Can you work these out from the model? Positions are in its coordinate system, mm. Face numbers are marked on the shaded views. A direction names the side the tool comes from. Coordinates: 2 decimals unless noted, no trailing zeros. Order: outer loops, then holes, each group sorted by start corner. A loop starts at its lowest first (then second) coordinate and runs counter-clockwise, first axis right, second up. Notation, with made-up numbers: (77, 11.5) -> (107, 11.5) arc R22 cw to (107, 36.5) -> close; hole circle Ø8 at (41.25, 20). An arc over 180 degrees is marked (long way). Write item = value, one per line.
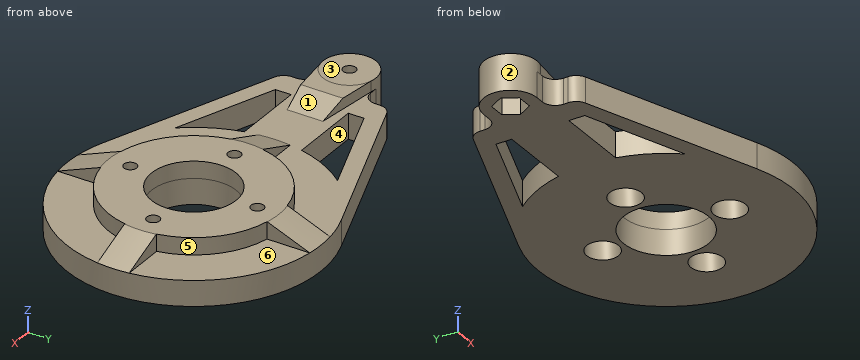
```python
from build123d import *
from OCP.BRepFilletAPI import BRepFilletAPI_MakeChamfer
from build123d.topology import SkipClean

# Parameters (mm, degrees)
SKETCH2_R           = 40
SKETCH2_R_2         = 20
BOSS_EXTRUDE1_DEPTH = 8
BOSS_EXTRUDE2_START = 12
SKETCH3_R           = 20
BOSS_EXTRUDE2_DEPTH = 12
SKETCH4_R           = 7.5
CUT_EXTRUDE1_DEPTH  = 10
SKETCH5_R           = 3
CUT_EXTRUDE2_DEPTH  = 29
BOSS_EXTRUDE3_DEPTH = 8
CHAMFER3_SIZE       = 8
CHAMFER3_SIZE_2     = 19.800694827
BOSS_EXTRUDE4_DEPTH = 12
FILLET1_R           = 6
CUT_EXTRUDE3_DEPTH  = 10
SKETCH9_R           = 3
CUT_EXTRUDE4_DEPTH  = 6
CUT_EXTRUDE5_START  = -22
CUT_EXTRUDE5_DEPTH  = 22
SKETCH12_R          = 12.5
SKETCH12_R_2        = 3
BOSS_EXTRUDE5_DEPTH = 5
BOSS_EXTRUDE6_DEPTH = 5
CHAMFER7_SIZE       = 8
CHAMFER7_SIZE_2     = 19.800694827


# Some blends are built 0.0001 mm under size
with BuildPart() as part:
    # Sketch2 → Boss-Extrude1 (new body)
    with BuildSketch(Plane.XY):
        Circle(SKETCH2_R)
        Circle(SKETCH2_R_2, mode=Mode.SUBTRACT)
    extrude(amount=BOSS_EXTRUDE1_DEPTH)

    # Sketch3 → Boss-Extrude2 (add)
    with SkipClean():  # the faces are left unmerged after this step: merging them gives an invalid solid
        with BuildSketch(Plane(origin=(0, 0, 0), x_dir=(-1, 0, 0), z_dir=(0, 0, -1)).offset(BOSS_EXTRUDE2_START)):
            with BuildLine():
                Line((105, -25), (105, 25))
                Line((105, 25), (20.894189842, 56.244402662))
                ThreePointArc((20.894189842, 56.244402662), (-60, 0), (20.894189842, -56.244402662))
                Line((20.894189842, -56.244402662), (105, -25))
            make_face()
            Circle(SKETCH3_R, mode=Mode.SUBTRACT)
        extrude(amount=-BOSS_EXTRUDE2_DEPTH)

    # Sketch4 → Cut-Extrude1 (cut)
    with SkipClean():  # the faces are left unmerged after this step: merging them gives an invalid solid
        with BuildSketch(Plane(origin=(0, 0, -12), x_dir=(-1, 0, 0), z_dir=(0, 0, -1))):
            with Locations((0, 30)):
                Circle(SKETCH4_R)
            with Locations((30, 0)):
                Circle(SKETCH4_R)
            with Locations((0, -30)):
                Circle(SKETCH4_R)
            with Locations((-30, 0)):
                Circle(SKETCH4_R)
        extrude(amount=-CUT_EXTRUDE1_DEPTH, mode=Mode.SUBTRACT)

    # Sketch5 → Cut-Extrude2 (cut)
    with SkipClean():  # the faces are left unmerged after this step: merging them gives an invalid solid
        with BuildSketch(Plane(origin=(0, 0, -2), x_dir=(-1, 0, 0), z_dir=(0, 0, -1))):
            with Locations((30, 0)):
                Circle(SKETCH5_R)
            with Locations((0, -30)):
                Circle(SKETCH5_R)
            with Locations((-30, 0)):
                Circle(SKETCH5_R)
            with Locations((0, 30)):
                Circle(SKETCH5_R)
        extrude(amount=-CUT_EXTRUDE2_DEPTH, mode=Mode.SUBTRACT)

    # Sketch6 → Boss-Extrude3 (add)
    with SkipClean():  # the faces are left unmerged after this step: merging them gives an invalid solid
        with BuildSketch(Plane.XY):
            with BuildLine():
                Line((39.290584114, -7.5), (59.529404499, -7.5))
                ThreePointArc((59.529404499, -7.5), (60, 0), (59.529404499, 7.5))
                Line((59.529404499, 7.5), (39.290584114, 7.5))
                ThreePointArc((39.290584114, 7.5), (40, 0), (39.290584114, -7.5))
            make_face()
            with BuildLine():
                Line((-7.5, 39.290584114), (-7.5, 59.529404499))
                ThreePointArc((-7.5, 59.529404499), (0, 60), (7.5, 59.529404499))
                Line((7.5, 59.529404499), (7.5, 39.290584114))
                ThreePointArc((7.5, 39.290584114), (0, 40), (-7.5, 39.290584114))
            make_face()
            with BuildLine():
                Line((-7.5, -39.290584114), (-7.5, -59.529404499))
                ThreePointArc((-7.5, -59.529404499), (0, -60), (7.5, -59.529404499))
                Line((7.5, -59.529404499), (7.5, -39.290584114))
                ThreePointArc((7.5, -39.290584114), (0, -40), (-7.5, -39.290584114))
            make_face()
            with BuildLine():
                Line((-39.290584114, 7.5), (-59.529404499, 7.5))
                ThreePointArc((-59.529404499, 7.5), (-60, 0), (-59.529404499, -7.5))
                Line((-59.529404499, -7.5), (-39.290584114, -7.5))
                ThreePointArc((-39.290584114, -7.5), (-40, 0), (-39.290584114, 7.5))
            make_face()
        extrude(amount=BOSS_EXTRUDE3_DEPTH)

    # Chamfer3
    chamfer3_edges_1 = [part.edges().sort_by_distance(p)[0] for p in [
        (0, 60, 8),
    ]]
    chamfer3_side_1 = [part.faces().sort_by_distance(p)[0] for p in [
        (0, 60, 7.84),
    ]]
    chamfer3_edges_2 = [part.edges().sort_by_distance(p)[0] for p in [
        (60, 0, 8),
    ]]
    chamfer3_side_2 = [part.faces().sort_by_distance(p)[0] for p in [
        (59.84, 0, 8),
    ]]
    chamfer3_edges_3 = [part.edges().sort_by_distance(p)[0] for p in [
        (-60, 0, 8),
    ]]
    chamfer3_side_3 = [part.faces().sort_by_distance(p)[0] for p in [
        (-59.84, 0, 8),
    ]]
    chamfer3_edges_4 = [part.edges().sort_by_distance(p)[0] for p in [
        (0, -60, 8),
    ]]
    chamfer3_side_4 = [part.faces().sort_by_distance(p)[0] for p in [
        (0, -59.84, 8),
    ]]
    chamfer3 = BRepFilletAPI_MakeChamfer(part.part.solid().wrapped)
    for e in chamfer3_edges_1:
        chamfer3.Add(CHAMFER3_SIZE - 0.0001, CHAMFER3_SIZE_2 - 0.0001, e.wrapped, chamfer3_side_1[0].wrapped)
    for e in chamfer3_edges_2:
        chamfer3.Add(CHAMFER3_SIZE_2 - 0.0001, CHAMFER3_SIZE - 0.0001, e.wrapped, chamfer3_side_2[0].wrapped)
    for e in chamfer3_edges_3:
        chamfer3.Add(CHAMFER3_SIZE_2 - 0.0001, CHAMFER3_SIZE - 0.0001, e.wrapped, chamfer3_side_3[0].wrapped)
    for e in chamfer3_edges_4:
        chamfer3.Add(CHAMFER3_SIZE_2 - 0.0001, CHAMFER3_SIZE - 0.0001, e.wrapped, chamfer3_side_4[0].wrapped)
    add(Compound.cast(chamfer3.Shape()), mode=Mode.REPLACE)  # a hair under: the kernel refuses the full size

    # Sketch7 → Boss-Extrude4 (add)
    with SkipClean():  # the faces are left unmerged after this step: merging them gives an invalid solid
        with BuildSketch(Plane(origin=(0, 0, -12), x_dir=(-1, 0, 0), z_dir=(0, 0, -1))):
            with BuildLine():
                Line((115, 12.5), (105, 12.5))
                Line((105, 12.5), (105, -12.5))
                Line((105, -12.5), (115, -12.5))
                ThreePointArc((115, -12.5), (127.5, 0), (115, 12.5))
            make_face()
        extrude(amount=-BOSS_EXTRUDE4_DEPTH)

    # Fillet1
    fillet1_edges = [part.edges().sort_by_distance(p)[0] for p in [
        (-105, -25, -6),
        (-105, 25, -6),
        (-105, -12.5, -6),
        (-105, 12.5, -6),
    ]]
    fillet(fillet1_edges, radius=FILLET1_R)

    # Sketch8 → Cut-Extrude3 (cut)
    with SkipClean():  # the faces are left unmerged after this step: merging them gives an invalid solid
        with BuildSketch(Plane(origin=(0, 0, -12), x_dir=(-1, 0, 0), z_dir=(0, 0, -1))):
            Polygon((118.778590974, 6.485027647), (111.2730968, 6.514869597), (107.494505826, 0.02984195), (111.221409026, -6.485027647), (118.7269032, -6.514869597), (122.505494174, -0.02984195), align=None)
        extrude(amount=-CUT_EXTRUDE3_DEPTH, mode=Mode.SUBTRACT)

    # Sketch9 → Cut-Extrude4 (cut)
    with SkipClean():  # the faces are left unmerged after this step: merging them gives an invalid solid
        with BuildSketch(Plane(origin=(0, 0, -2), x_dir=(-1, 0, 0), z_dir=(0, 0, -1))):
            with Locations((115, 0)):
                Circle(SKETCH9_R)
        extrude(amount=-CUT_EXTRUDE4_DEPTH, mode=Mode.SUBTRACT)

    # Sketch10 → Cut-Extrude5 (cut)
    with SkipClean():  # the faces are left unmerged after this step: merging them gives an invalid solid
        with BuildSketch(Plane.XY.offset(CUT_EXTRUDE5_START)):
            with BuildLine():
                Line((-58.46152581, -13.5), (-93, -13.5))
                Line((-93, -13.5), (-93, -20.923688206))
                Line((-93, -20.923688206), (-46.167935821, -38.321295672))
                ThreePointArc((-46.167935821, -38.321295672), (-53.766674065, -26.62977206), (-58.46152581, -13.5))
            make_face()
            with BuildLine():
                Line((-93, 20.923688206), (-46.167935821, 38.321295672))
                ThreePointArc((-46.167935821, 38.321295672), (-53.766674065, 26.62977206), (-58.46152581, 13.5))
                Line((-58.46152581, 13.5), (-93, 13.5))
                Line((-93, 13.5), (-93, 20.923688206))
            make_face()
        extrude(amount=CUT_EXTRUDE5_DEPTH, mode=Mode.SUBTRACT)

    # Sketch12 → Boss-Extrude5 (add)
    with SkipClean():  # the faces are left unmerged after this step: merging them gives an invalid solid
        with BuildSketch(Plane.XY):
            with Locations(Location((-115, 0, 0), (0, 0, 270))):
                Circle(SKETCH12_R)
            with Locations(Location((-115, 0, 0), (0, 0, 180))):
                Circle(SKETCH12_R_2, mode=Mode.SUBTRACT)
        extrude(amount=BOSS_EXTRUDE5_DEPTH)

    # Sketch13 → Boss-Extrude6 (add)
    with SkipClean():  # the faces are left unmerged after this step: merging them gives an invalid solid
        with BuildSketch(Plane.XY):
            with BuildLine():
                Line((-74.743265697, 7.5), (-112.037181998, 12.144415139))
                ThreePointArc((-112.037181998, 12.144415139), (-102.499395631, 0), (-112.037181998, -12.144415139))
                Line((-112.037181998, -12.144415139), (-74.743265697, -7.5))
                Line((-74.743265697, -7.5), (-74.743265697, 7.5))
            make_face()
        extrude(amount=BOSS_EXTRUDE6_DEPTH)

    # Chamfer7
    # the kernel refuses this chamfer: 19.800694827, 8 mm, written as the material it takes off along each edge
    with BuildSketch(Plane(origin=(-74.743265697, -58.842983777, 5), x_dir=(0.08816706473193492, 0, -0.9961057015681392), z_dir=(0, 1, 0))) as chamfer7_piece_1_section:
        Polygon((CHAMFER7_SIZE * 0.996105701568, CHAMFER7_SIZE * 0.0881670647319), (-CHAMFER7_SIZE_2 * 0.0881670647334, CHAMFER7_SIZE_2 * 0.996105701585), (0, 0), align=None)
    chamfer7_piece_1 = extrude(amount=117.685967554, mode=Mode.PRIVATE)
    chamfer7_piece_1 = split(chamfer7_piece_1, bisect_by=Plane(origin=(-82.305145915, 0, 0), z_dir=(0, 0, 1)), keep=Keep.TOP, mode=Mode.PRIVATE)
    add(chamfer7_piece_1, mode=Mode.SUBTRACT)


solid = part.part
```
Item 1: If we mould it in two halves opening along Y, with no side actions, what happens to the marked faces 4, 5 and 6? For each: pulls with the +Y half, pulls with the -Y half, needs draft (parallel to the pull), parting line crosses it, or undercut.
A:
face_4 = undercut
face_5 = pulls with the +Y half
face_6 = needs draft
Item 2: I want a section at C-C, the plane y = 30. Please give me the cut outline in (x, z).
A:
outline = (-91.54, -12) -> (-68.57, -12) -> (-68.57, 0) -> (-91.54, 0) -> close; (-51.96, -12) -> (-7.5, -12) -> (-7.5, -2) -> (-3, -2) -> (-3, 8) -> (-26.46, 8) -> (-26.46, 0) -> (-51.96, 0) -> close; (3, -2) -> (7.5, -2) -> (7.5, -12) -> (51.96, -12) -> (51.96, 0) -> (26.46, 0) -> (26.46, 8) -> (3, 8) -> close
Item 3: If I drill on probe 1 along Y at (x, z) = (0, 3.5); probe 2 along Y at (x, z) = (-30, 3); probe 3 along Y at (x, z) = (1, 5), over which ranges is the centre line in solid material (lowest first)?
A:
probe_1 = -51.34 to -33, -27 to -20, 20 to 27, 33 to 51.34
probe_2 = -26.46 to -3, 3 to 26.46
probe_3 = -47.61 to -32.83, -27.17 to -19.97, 19.97 to 27.17, 32.83 to 47.61
Item 4: I want a section at A-A, the plane z = -6.75. Give the number of separate pieces and of enclosed holes in the cut face, plus the area to 3 significant figures.
A:
separate_pieces = 1
enclosed_holes = 8
area = 12,200 mm2
Item 5: I'm going to push flat-ended pins straight in: P1, Ø1, axis at x = -23.5, z = -6.5, coming from the -Y side; P2, Ø10, axis at x = 39, z = 1.5, coming from the -Y side; P3, Ø2.5, axis at y = -45, z = 5, coming from the -X side; P4, Ø14.5, axis at x = -112, y = -1.5, coming from the -Z side. Where does each tip first touch, or does it pass through?
A:
P1 = -55.46
P2 = -49.28
P3 = -7.5
P4 = -12
Item 6: I want a section at D-D, the plane x = -63.5. Please give me the cut outline in (y, z), plus the area to 3 significant figures.
A:
outline = (-40.42, -12) -> (-31.88, -12) -> (-31.88, 0) -> (-40.42, 0) -> close; (-13.5, -12) -> (13.5, -12) -> (13.5, 0) -> (-13.5, 0) -> close; (31.88, -12) -> (40.42, -12) -> (40.42, 0) -> (31.88, 0) -> close
area = 529 mm2
Item 7: I want a section at B-B, the plane x = -30. Please give me the cut outline in (y, z), plus the area to 3 significant figures.
A:
outline = (-52.86, -12) -> (-7.5, -12) -> (-7.5, -2) -> (-3, -2) -> (-3, 8) -> (-26.46, 8) -> (-26.46, 0) -> (-52.86, 0) -> close; (3, -2) -> (7.5, -2) -> (7.5, -12) -> (52.86, -12) -> (52.86, 0) -> (26.46, 0) -> (26.46, 8) -> (3, 8) -> close
area = 1,480 mm2
Item 8: For the marked faces 1, 2 and 3, which set-ups out of +Z, -Z, +X, -X, +Y, -Y let a thin tool reach every point of the face, with its end or its side?
A:
face_1 = +Z, +Y, -Y
face_2 = none
face_3 = +Z, -X, +Y, -Y
